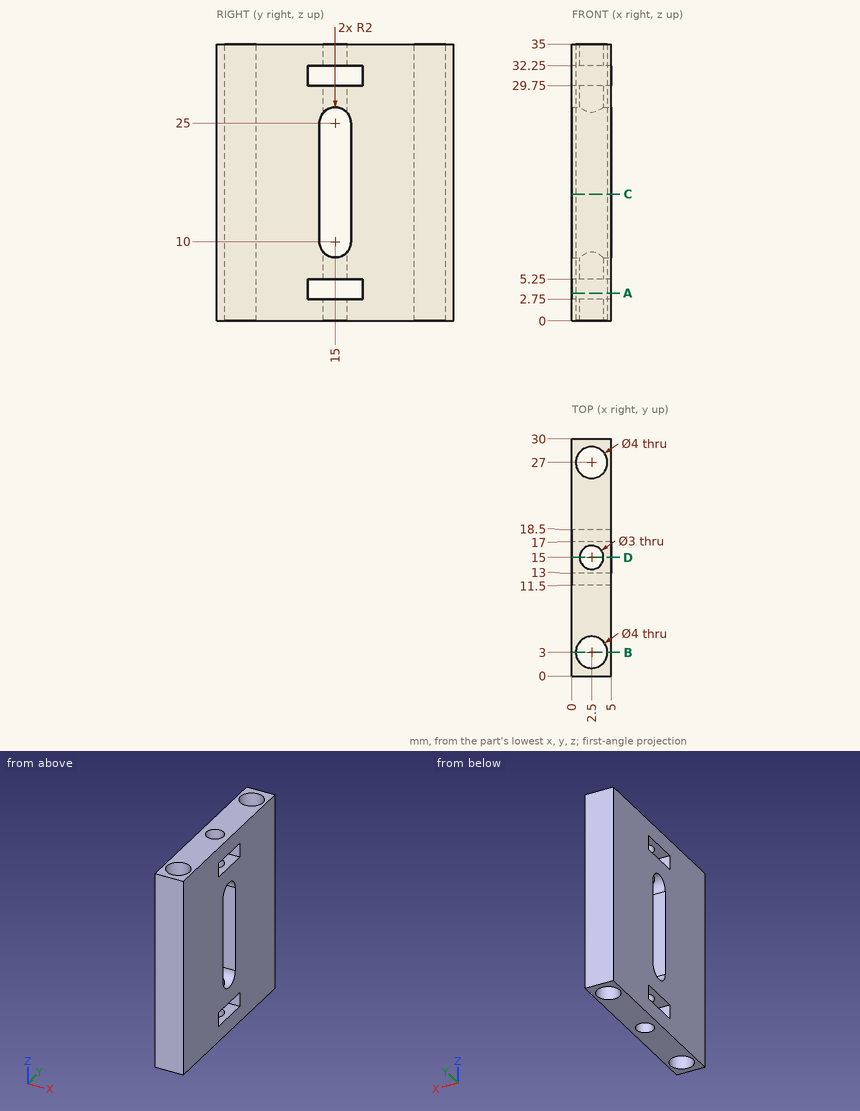
Geometry check sheet. Reference: drawing and pictorial views, mm from the part's lowest x, y, z. Coordinates: 2 decimals unless noted, no trailing zeros. Order: outer loops, then holes, each group sorted by start corner. A loop starts at its lowest first (then second) coordinate and runs counter-clockwise, first axis right, second up.
Item 1: Section check C-C (z = 16). Enter the section's corners in (x, y).
Item 2: Section check D-D (y = 15). Count the separate pieces of the cut face and the enclosed holes in it, plus the area to 3 significant figures.
Item 3: Section check B-B (y = 3). Enter the section's corners in (x, z), plus the area to 3 significant figures.
Item 4: Section check A-A (z = 3.5). Enter the section's corners in (x, y).
Item 5: Depth check by flat-ended pin: pin 1 (2.5 mm diameter, centred on x = 2.5, y = 15, fed in from -Z). Enter the tip coordinate at first touch or a pass-through.
Item 6: Scan lines: line 1 along Y through (x, z) = (2.5, 7.1); line 2 along Y through (x, z) = (2.4, 3); line 3 along Z through (x, y) = (4.15, 13.5). Record each from-to range of solid material in increasing order.
Check sheet entries:
1. outline: (0, 0) - (5, 0) - (5, 13) - (0, 13) - close; (0, 17) - (5, 17) - (5, 30) - (0, 30) - close; hole circle Ø4 at (2.5, 3); hole circle Ø4 at (2.5, 27)
2. separate pieces: 8
2. enclosed holes: 0
2. area: 22.0 mm2
3. outline: (0, 0) - (0.5, 0) - (0.5, 35) - (0, 35) - close; (4.5, 0) - (5, 0) - (5, 35) - (4.5, 35) - close
3. area: 35.0 mm2
4. outline: (0, 0) - (5, 0) - (5, 11.5) - (0, 11.5) - close; (0, 18.5) - (5, 18.5) - (5, 30) - (0, 30) - close; hole circle Ø4 at (2.5, 3); hole circle Ø4 at (2.5, 27)
5. pin 1: passes through
6. line 1: y = 0 to 1, 5 to 13.5, 16.5 to 25, 29 to 30
6. line 2: y = 0 to 1, 5 to 11.5, 18.5 to 25, 29 to 30
6. line 3: z = 0 to 2.75, 5.25 to 8.68, 26.32 to 29.75, 32.25 to 35
